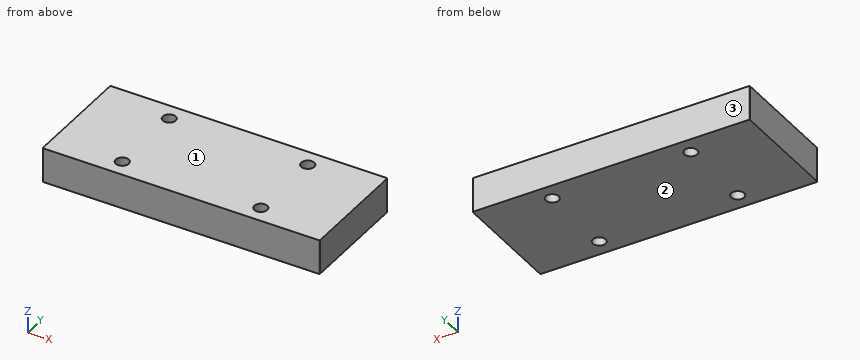
from build123d import *

# Parameters (mm, degrees)
F0_R     = 4.7625
F1_DEPTH = 25.4


with BuildPart() as f1:
    # F0 (on Top) → F1 (new body)
    with BuildSketch(Plane.XY):
        with BuildLine():
            Line((151.638, 12.7), (-50.038, 12.7))
            ThreePointArc((-50.038, 12.7), (-50.576815, 12.476815), (-50.8, 11.938))
            Line((-50.8, 11.938), (-50.8, -69.088))
            ThreePointArc((-50.8, -69.088), (-50.576815, -69.626815), (-50.038, -69.85))
            Line((-50.038, -69.85), (151.638, -69.85))
            ThreePointArc((151.638, -69.85), (152.176815, -69.626815), (152.4, -69.088))
            Line((152.4, -69.088), (152.4, 11.938))
            ThreePointArc((152.4, 11.938), (152.176815, 12.476815), (151.638, 12.7))
        make_face()
        with Locations((0, -57.15)):
            Circle(F0_R, mode=Mode.SUBTRACT)
        with Locations((101.6, -57.15)):
            Circle(F0_R, mode=Mode.SUBTRACT)
        Circle(F0_R, mode=Mode.SUBTRACT)
        with Locations((101.6, 0)):
            Circle(F0_R, mode=Mode.SUBTRACT)
    extrude(amount=F1_DEPTH)


solid = f1.part
Model file for the job. Use its own axes, mm. Face numbers are marked on the shaded views. Give positions to 0.01 mm unless a question says otherwise; leave off trailing zeros. Order: outer loops, then holes, each group sorted by start corner. A loop starts at its lowest first (then second) coordinate and runs counter-clockwise, first axis right, second up. Notation, with made-up numbers: (19.5, 26.25) - (49.5, 26.25) arc R28 ccw to (49.5, 60.25) - close; hole circle Ø9 at (87, -34.75). An arc over 180 degrees is marked (long way). One line per item, written item: value.
Item 1: Slice it at C-C (z = 18). Give the number of separate pieces and of enclosed holes in the cut face, then the cut area to 3 significant figures.
Response values:
separate pieces: 1
enclosed holes: 4
area: 16,500 mm2
Item 2: Wall check: line 1 (Y direction, x = 101.6, z = 19.25); line 2 (X direction, y = -59.5, z = 14.5); line 3 (Y direction, x = 2, z = 6.25). Give the ranges that are in metal, low to high.
Response values:
line 1: -69.85 to -61.91, -52.39 to -4.76, 4.76 to 12.7
line 2: -50.8 to -4.14, 4.14 to 97.46, 105.74 to 152.4
line 3: -69.85 to -61.47, -52.83 to -4.32, 4.32 to 12.7
Item 3: Slice it at A-A (y = -57.15). List the corners of the cut face in (x, z), then the cut area to 3 significant figures.
Response values:
outline: (-50.8, 0) - (-4.76, 0) - (-4.76, 25.4) - (-50.8, 25.4) - close; (4.76, 0) - (96.84, 0) - (96.84, 25.4) - (4.76, 25.4) - close; (106.36, 0) - (152.4, 0) - (152.4, 25.4) - (106.36, 25.4) - close
area: 4,680 mm2
Item 4: Two-plate mould, pull along Z, no slides. Class the marked faces 1, 2 and 3: released by +Z, released by -Z, zero draft, split by the parting line, or undercut.
Response values:
face 1: released by +Z
face 2: released by -Z
face 3: zero draft
Item 5: Pin check, flat tips, straight feed: pin 1 Ø5.5 at (x, y) = (101.6, 0) entering from -Z; pin 2 Ø12.5 at (x, y) = (0, 0) entering from +Z. Stop position of each tip, or through.
Response values:
pin 1: through
pin 2: z = 25.4
Item 6: Slice it at B-B (x = 101.6). List the corners of the cut face in (y, z).
Response values:
outline: (-69.85, 0) - (-61.91, 0) - (-61.91, 25.4) - (-69.85, 25.4) - close; (-52.39, 0) - (-4.76, 0) - (-4.76, 25.4) - (-52.39, 25.4) - close; (4.76, 0) - (12.7, 0) - (12.7, 25.4) - (4.76, 25.4) - close
